Verification items for the finished model (mm, model axes). Face numbers are marked on the shaded views. Round coordinates to 2 decimals unless told otherwise and drop trailing zeros. Write each loop counter-clockwise with the first axis right and the second up, starting at its lowest first coordinate (ties: lowest second). Pieces come first, ordered by that corner, then holes. Notation, with made-up numbers: M 38,-28 L 70,-28 A25 ccw 70,5 Z; hole C 52.25,29.25 d9. An arc over 180 degrees is marked long. Write each question's results on one line, items separated by ' | '.
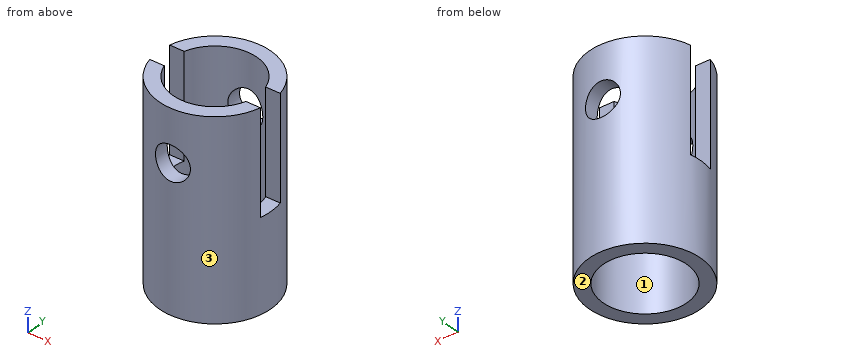
from build123d import *

# Parameters (mm, degrees)
F0_R          = 24.4
F0_R_2        = 18.36585117
F1_DEPTH      = 60
F2_R          = 24.4
F2_R_2        = 18.36585117
F3_DEPTH      = 25
F5_DEPTH      = 24.401
F5_DEPTH_BACK = 24.401
F6_R          = 7.5
F7_DEPTH      = 24.401
F7_DEPTH_BACK = 24.401


with BuildPart() as f1:
    # F0 (on Top) → F1 (new body)
    with BuildSketch(Plane.XY):
        Circle(F0_R)
        Circle(F0_R_2, mode=Mode.SUBTRACT)
    extrude(amount=F1_DEPTH)

    # F2 (on Top) → F3 (join)
    with BuildSketch(Plane.XY):
        Circle(F2_R)
        Circle(F2_R_2, mode=Mode.SUBTRACT)
    extrude(amount=-F3_DEPTH)

    # F4 (on Right) → F5 (cut, two sides)
    with BuildSketch(Plane.YZ) as f5_sk:
        Polygon((5.5, 60), (0, 60), (-5.5, 60), (-5.5, 15), (0, 15), (5.5, 15), align=None)
    extrude(amount=-F5_DEPTH, mode=Mode.SUBTRACT)
    extrude(f5_sk.sketch, amount=F5_DEPTH_BACK, mode=Mode.SUBTRACT)

    # F6 (on Front) → F7 (cut, two sides)
    with BuildSketch(Plane.XZ) as f7_sk:
        with Locations((0, 37.5)):
            Circle(F6_R)
    extrude(amount=-F7_DEPTH, mode=Mode.SUBTRACT)
    extrude(f7_sk.sketch, amount=F7_DEPTH_BACK, mode=Mode.SUBTRACT)


solid = f1.part
1) Sectioned sample at D-D, the plane x = -16. Record the cut outline in (y, z).
Calculated:
outline: M -18.42,-25 L -9.02,-25 L -9.02,60 L -18.42,60 Z; M 9.02,-25 L 18.42,-25 L 18.42,60 L 9.02,60 Z
2) Depth check by flat-ended pin: P1, Ø1.9, axis at x = 21, z = 34.5, coming from the -Y side; P2, Ø4, axis at x = 12, z = 23.5, coming from the +Y side; P3, Ø1.5, axis at y = 6.5, z = -4, coming from the +X side. Enter the tip coordinate at first touch or a pass-through.
Calculated:
P1: stops at y = -13.91 | P2: stops at y = 22.26 | P3: stops at x = 23.71
3) Draft check along Y on the marked faces 1, 2 and 3. Enter one of: pulls with the +Y half, pulls with the -Y half, needs draft (parallel to the pull), parting line crosses it, or undercut.
Calculated:
face 1: undercut | face 2: needs draft | face 3: parting line crosses it
4) Material ranges on line 1 (Y direction, x = 0, z = -2.5); line 2 (Z direction, x = 0, y = 21); line 3 (Z direction, x = -19, y = -1), recorded low to high. Write a range as [from, to].
Calculated:
line 1: y = [-24.4, -18.37], [18.37, 24.4] | line 2: z = [-25, 30], [45, 60] | line 3: z = [-25, 15]
5) Sectioned sample at B-B, the plane z = 37.5. Record the cut outline in (x, y).
Calculated:
outline: M -23.77,-5.5 A24.4 ccw -7.5,-23.22 L -7.5,-16.76 A18.37 cw -17.52,-5.5 Z; M -23.77,5.5 L -17.52,5.5 A18.37 cw -7.5,16.76 L -7.5,23.22 A24.4 ccw Z; M 7.5,-23.22 A24.4 ccw 23.77,-5.5 L 17.52,-5.5 A18.37 cw 7.5,-16.76 Z; M 7.5,16.76 A18.37 cw 17.52,5.5 L 23.77,5.5 A24.4 ccw 7.5,23.22 Z
6) Sectioned sample at C-C, the plane y = 0. Record the cut outline in (x, z).
Calculated:
outline: M -24.4,-25 L -18.37,-25 L -18.37,15 L -24.4,15 Z; M 18.37,-25 L 24.4,-25 L 24.4,15 L 18.37,15 Z
7) Sectioned sample at A-A, the plane x = 0. Record the cut outline in (y, z).
Calculated:
outline: M -24.4,-25 L -18.37,-25 L -18.37,30 L -24.4,30 Z; M -24.4,45 L -18.37,45 L -18.37,60 L -24.4,60 Z; M 18.37,-25 L 24.4,-25 L 24.4,30 L 18.37,30 Z; M 18.37,45 L 24.4,45 L 24.4,60 L 18.37,60 Z
